Input: part model. Units: mm. Frame: model coordinates. A direction names the side the tool comes from. Coordinates: 2 decimals unless noted, no trailing zeros. Write each loop counter-clockwise with the first axis right and the second up, starting at its lowest first coordinate (ties: lowest second). Pieces come first, ordered by that corner, then holes. Notation, with made-up numbers: (63.25, 63) - (74.25, 63) arc R16 ccw to (74.25, 80) - close; hole circle Ø9 at (43.25, 14). An arc over 180 degrees is marked (long way). Put each result on its own line as item: value. Start each with the question number.
1. Line query: line 1 (Y direction, x = 0, z = 1.35); line 2 (Z direction, x = 19.5, y = -8); line 3 (Y direction, x = 25, z = 5.7). Output: solid intervals per line, ascending.
2. Pull-direction query (X, two-part tool) for faces 3 (the flat face through (0, -28.817, 3)), 4 (the cylindrical face through (20.09, 14.14, 4.48)), 5 (the cylindrical face through (-25.271, -21.316, 2.958)); classes: released by +X, released by -X, zero draft, split by the parting line, or undercut.
3. Pin query (flat end, axial travel): pin 1 (3 mm diameter, centred on y = 5, z = 2.5, fed in from -X); pin 2 (3 mm diameter, centred on y = 13.5, z = 0.5, fed in from -X). Return the tip coordinate at first contact, or that it passes through.
4. Access query for faces 1 (the flat face through (0, 19.621, 4)), 2 (the cylindrical face through (25.271, 19.382, 2.958)). Directions: +Z, -Z, +X, -X, +Y, -Y. A direction counts if a zero-diameter tool reaches every point of the face in a straight line with its end or side. Return the directions, or none.
5. Cut plane C-C, the plane y = 2.5. Return loops of the section in (x, z).
6. Cut plane A-A, the plane z = 0.95. Return loops of the section in (x, y), and give its area (3 significant figures).
7. Cut plane B-B, the plane x = 0. Return loops of the section in (y, z).
8. Cut plane D-D, the plane x = 21.5. Return loops of the section in (y, z).
Autodesk Inventor part; units mm, degrees
ref_plane "YZ Plane" through (0, 0, 0) normal (1, 0, 0) x (0, 1, 0)
ref_plane "XZ Plane" through (0, 0, 0) normal (0, 1, 0) x (-1, 0, 0)
ref_plane "XY Plane" through (0, 0, 0) normal (0, 0, 1) x (1, 0, 0)
sketch "Sketch1" plane through (0, 0, 0) normal (0, 0, 1) x (1, 0, 0)
  line L0 (-40, 40) -> (40, 40)
  line L1 (40, 40) -> (40, -40)
  line L2 (40, -40) -> (-40, -40)
  line L3 (-40, -40) -> (-40, 40)
  line L4 (-40, 40) -> (40, -40) construction
  line L5 (40, 40) -> (-40, -40) construction
  point P0 (0, 0)
  dimension "d0" = 80
  dimension "d1" = 80
extrude "Extrusion1" add sketch "Sketch1" along normal blind 3
sketch "Sketch2" plane through (0, 0, 3) normal (0, 0, 1) x (1, 0, 0)
  arc A0 (-2, 26.8827) -> (-40, -0.967) centre (-2, -12.967) ccw
  arc A1 (40, -0.967) -> (2, 26.8827) centre (2, -12.967) ccw
  line L0 (2, 26.8827) -> (-2, 26.8827)
  line L1 (-40, -0.967) -> (40, -0.967) construction
  line L2 (40, -40) -> (40, 40) construction
  arc A2 (-2, 26.8827) -> (-40, -0.967) centre (-2, -12.967) ccw construction
  arc A3 (40, -0.967) -> (2, 26.8827) centre (2, -12.967) ccw construction
  arc A4 (-2, 26.8827) -> (-40, -0.967) centre (-2, -12.967) ccw
  arc A5 (40, -0.967) -> (2, 26.8827) centre (2, -12.967) ccw
  line L3 (-2, 26.8827) -> (2, 26.8827)
  arc A6 (-2, 26.8827) -> (-40, -0.967) centre (-2, -12.967) ccw
  arc A7 (40, -0.967) -> (2, 26.8827) centre (2, -12.967) ccw
  line L4 (2, 26.8827) -> (-2, 26.8827)
  arc A8 (-40, -0.967) -> (-2, -28.8167) centre (-2, 11.033) ccw
  arc A9 (2, -28.8167) -> (40, -0.967) centre (2, 11.033) ccw
  line L5 (2, -28.8167) -> (-2, -28.8167)
  line L6 (-40, 40) -> (-40, -40)
  line L7 (-40, -0.967) -> (-40, 40)
  line L8 (40, 40) -> (-40, 40)
  line L9 (-40, 40) -> (40, 40)
  line L10 (40, 40) -> (40, -0.967)
  line L11 (40, -0.967) -> (40, -40)
  line L12 (-40, -40) -> (40, -40)
  line L13 (-40, -40) -> (40, -40)
  line L14 (40, -40) -> (-40, -40)
  point P0 (0, 0)
extrude "Extrusion2" cut sketch "Sketch2" against normal blind 3 contours A0 L6 L8 L10 A1 L0 | A8 L5 A9 L11 L12 L6
sketch "Sketch3" plane through (0, 0, 3) normal (0, 0, 1) x (1, 0, 0)
  circle A0 centre (0, -0.967) radius 16
  point P0 (0, 0)
extrude "Extrusion3" cut sketch "Sketch3" against normal blind 3
sketch "Sketch4" plane through (0, 0, 3) normal (0, 0, 1) x (1, 0, 0)
  arc A0 (-2, 19.6211) -> (-32.2982, -0.967) centre (-2, -12.967) ccw
  arc A1 (32.2982, -0.967) -> (2, 19.6211) centre (2, -12.967) ccw
  line L0 (-2, 19.6211) -> (2, 19.6211)
  arc A2 (-2, 19.6211) -> (-32.2982, -0.967) centre (-2, -12.967) ccw
  arc A3 (32.2982, -0.967) -> (2, 19.6211) centre (2, -12.967) ccw
  line L1 (2, 19.6211) -> (-2, 19.6211)
  line L2 (32.2982, -0.967) -> (-32.2982, -0.967) construction
  arc A4 (-32.2982, -0.967) -> (-2, -21.5551) centre (-2, 11.033) ccw
  arc A5 (2, -21.5551) -> (32.2982, -0.967) centre (2, 11.033) ccw
  line L3 (-2, -21.5551) -> (2, -21.5551)
  arc A6 (-2, 26.8827) -> (-40, -0.967) centre (-2, -12.967) ccw construction
  line L4 (-2, 26.8827) -> (2, 26.8827) construction
  arc A7 (40, -0.967) -> (2, 26.8827) centre (2, -12.967) ccw construction
  arc A8 (-40, -0.967) -> (-2, -28.8167) centre (-2, 11.033) ccw construction
  line L5 (2, -28.8167) -> (-2, -28.8167) construction
  arc A9 (2, -28.8167) -> (35, -11.3053) centre (2, 11.033) ccw construction
  arc A10 (2, -28.8167) -> (40, -0.967) centre (2, 11.033) ccw construction
  arc A11 (-2, 26.8827) -> (-40, -0.967) centre (-2, -12.967) ccw construction
  arc A12 (-2, 26.8827) -> (-40, -0.967) centre (-2, -12.967) ccw
  arc A13 (40, -0.967) -> (2, 26.8827) centre (2, -12.967) ccw
  arc A14 (2, -28.8167) -> (40, -0.967) centre (2, 11.033) ccw
  arc A15 (-40, -0.967) -> (-2, -28.8167) centre (-2, 11.033) ccw
  line L6 (-2, 26.8827) -> (2, 26.8827)
  line L7 (-2, 26.8827) -> (2, 26.8827)
  line L8 (2, -28.8167) -> (-2, -28.8167)
  point P0 (0, 0)
extrude "Extrusion4" add sketch "Sketch4" along normal blind 3
Report:
1. line 1: y = -28.82 to -16.97, 15.03 to 26.88
1. line 2: z = 0 to 3
1. line 3: y = -21.51 to -12.05, 10.12 to 19.58
2. face 3: zero draft
2. face 4: undercut
2. face 5: released by -X
3. pin 1: stops at x = -38.29
3. pin 2: stops at x = -33.06
4. face 1: +Z
4. face 2: +Z, -Z, +X, +Y
5. outline: (-38.73, 0) - (-15.62, 0) - (-15.62, 3) - (-30.68, 3) - (-30.68, 6) - (-38.73, 6) - close; (15.62, 0) - (38.73, 0) - (38.73, 6) - (30.68, 6) - (30.68, 3) - (15.62, 3) - close
6. outline: (-40, -0.97) arc R39.85 ccw to (-2, -28.82) - (2, -28.82) arc R39.85 ccw to (40, -0.97) arc R39.85 ccw to (2, 26.88) - (-2, 26.88) arc R39.85 ccw to start; hole circle Ø32 at (0, -0.97)
6. area: 2,520 mm^2
7. outline: (-28.82, 0) - (-16.97, 0) - (-16.97, 3) - (-21.56, 3) - (-21.56, 6) - (-28.82, 6) - close; (15.03, 0) - (26.88, 0) - (26.88, 6) - (19.62, 6) - (19.62, 3) - (15.03, 3) - close
8. outline: (-23.72, 0) - (21.79, 0) - (21.79, 6) - (13.14, 6) - (13.14, 3) - (-15.08, 3) - (-15.08, 6) - (-23.72, 6) - close
